Verification items for the finished model (mm, model axes). A direction names the side the tool comes from. Give positions to 0.01 mm unless a question says otherwise; leave off trailing zeros. Order: outer loops, then holes, each group sorted by start corner. A loop starts at its lowest first (then second) coordinate and runs counter-clockwise, first axis right, second up. Notation, with made-up numbers: (10, 22.5) - (14, 22.5) arc R22 ccw to (14, 32.5) - close; hole circle Ø5 at (-5.75, 71). An arc over 180 degrees is marked (long way). Answer as a JSON object with one key per item and string values. Group by question number.
(1) Section check B-B (z = -35). Record the boundary of the cut face in (x, y), then the cut area to 3 significant figures.
(2) Mould release check, pull along Z, two halves, no side actions. Record for faces 4 (the face through (21, 103, -36)), 5 (the face through (19.3, 105.2, -40.25)), 6 (the face through (19.3, 105.2, 31.75)): +Z half, -Z half, draft (parallel to the pull), parting line (faces both ways), or undercut.
(3) Section check A-A (x = 16). Record the boundary of the cut face in (y, z), then the cut area to 3 significant figures.
(4) Depth check by flat-ended pin: pin 1 Ø4.5 at (y, z) = (102, 36.5) entering from -X; pin 2 Ø2.5 at (y, z) = (104, -36.5) entering from +X; pin 3 Ø1.2 at (y, z) = (103.5, -38) entering from -X; pin 4 Ø3 at (x, z) = (-10.5, 15.5) entering from +Y. Enter the tip coordinate at first touch or a pass-through.
(5) Section check D-D (z = -19). Record the boundary of the cut face in (x, y).
(6) Thickness scan on line 1 (Y direction, x = -22, z = 3.5); line 2 (Y direction, x = 18, z = 36). Record the ranges inside material, lowest first.
(7) Access from +Z, -Z, +X, -X, +Y, -Y to the whole of each face (thin tool, end or side, straight path). Record for faces 1 (the face through (22, 103, -36)), 2 (the face through (19.3, 105.2, 40.25)), 3 (the face through (19.3, 105.2, -31.75)).
(8) Section check C-C (x = -27). Record the boundary of the cut face in (y, z).
```python
from build123d import *

# Parameters (mm, degrees)
SKETCH_2_W          = 70
SKETCH_2_H          = 90
EXTRUDE_1_DEPTH     = 101
SKETCH_3_W          = 7.5
SKETCH_3_H          = 8.5
EXTRUDE_1_2_DEPTH   = 5
SKETCH_4_W          = 6.5
SKETCH_4_H          = 4
CUT_EXTRUDE_1_DEPTH = 141.458401315


with BuildPart() as part:
    # 草图2 → Extrude 1 (new body)
    with BuildSketch(Plane(origin=(0, 0, 0), x_dir=(1, 0, 0), z_dir=(0, 1, 0))):
        Rectangle(SKETCH_2_W, SKETCH_2_H)
    extrude(amount=EXTRUDE_1_DEPTH)

    # 草图3 → Extrude 1 2 (add)
    with BuildSketch(Plane(origin=(0, 101, 0), x_dir=(1, 0, 0), z_dir=(0, 1, 0))):
        with Locations((18.25, 36)):
            Rectangle(SKETCH_3_W, SKETCH_3_H)
        with Locations((18.25, -36)):
            Rectangle(SKETCH_3_W, SKETCH_3_H)
    extrude(amount=EXTRUDE_1_2_DEPTH)

    # 草图4 → 切除-拉伸1 (cut, through all)
    with BuildSketch(Plane.XY.offset(40.25)):
        with Locations((17.75, 103)):
            Rectangle(SKETCH_4_W, SKETCH_4_H)
    extrude(amount=-CUT_EXTRUDE_1_DEPTH, mode=Mode.SUBTRACT)


solid = part.part
```
Solutions:
{
 "1": {"outline": "(-35, 0) - (35, 0) - (35, 101) - (22, 101) - (22, 106) - (14.5, 106) - (14.5, 105) - (21, 105) - (21, 101) - (-35, 101) - close", "area": "7,080 mm2"},
 "2": {"face 4": "draft", "face 5": "-Z half", "face 6": "undercut"},
 "3": {"outline": "(0, -45) - (101, -45) - (101, 45) - (0, 45) - close; (105, -40.25) - (106, -40.25) - (106, -31.75) - (105, -31.75) - close; (105, 31.75) - (106, 31.75) - (106, 40.25) - (105, 40.25) - close", "area": "9,110 mm2"},
 "4": {"pin 1": "stops at x = -35", "pin 2": "stops at x = 22", "pin 3": "stops at x = 21", "pin 4": "stops at y = 101"},
 "5": {"outline": "(-35, 0) - (35, 0) - (35, 101) - (-35, 101) - close"},
 "6": {"line 1": "y = 0 to 101", "line 2": "y = 0 to 101, 105 to 106"},
 "7": {"face 1": "+Z, -Z, +X, +Y", "face 2": "+Z, +X, -X, +Y", "face 3": "+X, -X, +Y"},
 "8": {"outline": "(0, -45) - (101, -45) - (101, 45) - (0, 45) - close"}
}
